from build123d import *

# Parameters (mm, degrees)
F0_W     = 20
F0_H     = 10.1
F1_DEPTH = 1.5
F2_R     = 1.1
F3_DEPTH = 1.5
F4_R     = 1


with BuildPart() as f1:
    # F0 (on Front) → F1 (new body)
    with BuildSketch(Plane.XZ):
        with Locations((10, 5.05)):
            Rectangle(F0_W, F0_H)
    extrude(amount=F1_DEPTH)

    # F2 (on face) → F3 (cut, through all)
    with BuildSketch(Plane.XZ.offset(1.5)):
        with Locations((2.3, 7.9)):
            Circle(F2_R)
        with Locations((17.7, 7.9)):
            Circle(F2_R)
        with Locations((2.3, 2.2)):
            Circle(F2_R)
        with Locations((17.7, 2.2)):
            Circle(F2_R)
        with BuildLine():
            Line((15.123475383, 10.1), (4.876524617, 10.1))
            ThreePointArc((4.876524617, 10.1), (10, 7.6), (15.123475383, 10.1))
        make_face()
        with BuildLine():
            ThreePointArc((15.123475383, 0), (10, 2.5), (4.876524617, 0))
            Line((4.876524617, 0), (15.123475383, 0))
        make_face()
    extrude(amount=-F3_DEPTH, mode=Mode.SUBTRACT)

    # F4
    f4_edges = [f1.edges().sort_by_distance(p)[0] for p in [
        (20, -0.75, 10.1),
        (20, -0.75, 0),
        (0, -0.75, 10.1),
        (0, -0.75, 0),
        (4.876525, -0.75, 10.1),
        (15.123475, -0.75, 10.1),
        (4.876525, -0.75, 0),
        (15.123475, -0.75, 0),
    ]]
    fillet(f4_edges, radius=F4_R)


solid = f1.part
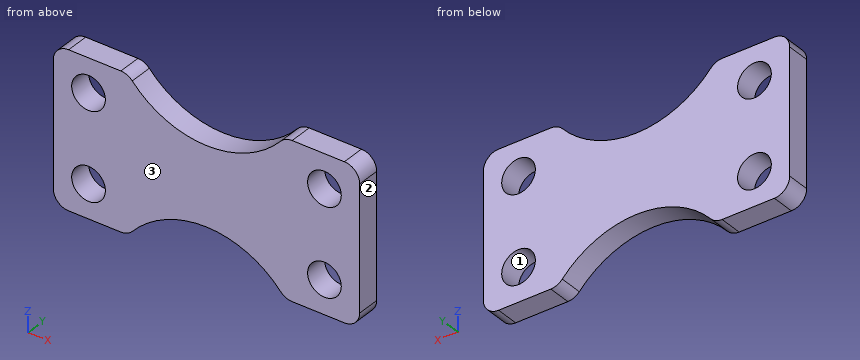
For this review, take the finished solid that the model builds, in its own axes (mm). Face numbers are marked on the shaded views. Give positions to 0.01 mm unless a question says otherwise; leave off trailing zeros. Order: outer loops, then holes, each group sorted by start corner. A loop starts at its lowest first (then second) coordinate and runs counter-clockwise, first axis right, second up. Notation, with made-up numbers: (13.5, 71.5) - (30.5, 71.5) arc R16 cw to (30.5, 83.5) - close; hole circle Ø3 at (37.5, 51). An arc over 180 degrees is marked (long way). Answer as a JSON object with one key per item and string values. Group by question number.
Item 1: Take a section at D-D on z = 7. Give the boundary of the cut face in (x, y), and give its area (3 significant figures).
Item 2: Take a section at B-B on z = 8.25. Give the boundary of the cut face in (x, y), and give its area (3 significant figures).
Item 3: Draft analysis for pull direction X (two halves, no side actions). For the marked faces 1, 2 and 3, state which applies: pulls with the +X half, pulls with the -X half, needs draft (parallel to the pull), parting line crosses it, or undercut.
Item 4: Take a section at A-A on x = 2.3. Give the boundary of the cut face in (y, z).
Item 5: Take a section at C-C on y = -1.15. Give the boundary of the cut face in (x, z).
Item 6: Wall thickness on line 1 along Z through (x, y) = (17.7, -1.2); line 2 along X through (y, z) = (-0.65, 2); line 3 along X through (y, z) = (-0.7, 1.5): over which ranges is each line inside the solid? List them lowest first.
Item 7: Clearance check with a flat-ended pin moving along its axis: pin 1 Ø2.5 at (x, z) = (17.7, 7.9) entering from +Y. State where the tip first meets the part, or that it passes through.
Reported:
{
 "1": {"outline": "(0, -1.5) - (1.67, -1.5) - (1.67, 0) - (0, 0) - close; (2.93, -1.5) - (17.07, -1.5) - (17.07, 0) - (2.93, 0) - close; (18.33, -1.5) - (20, -1.5) - (20, 0) - (18.33, 0) - close", "area": "26.2 mm^2"},
 "2": {"outline": "(0, -1.5) - (1.26, -1.5) - (1.26, 0) - (0, 0) - close; (3.34, -1.5) - (7.17, -1.5) - (7.17, 0) - (3.34, 0) - close; (12.83, -1.5) - (16.66, -1.5) - (16.66, 0) - (12.83, 0) - close; (18.74, -1.5) - (20, -1.5) - (20, 0) - (18.74, 0) - close", "area": "15.2 mm^2"},
 "3": {"face 1": "undercut", "face 2": "pulls with the +X half", "face 3": "needs draft"},
 "4": {"outline": "(-1.5, 0) - (0, 0) - (0, 1.1) - (-1.5, 1.1) - close; (-1.5, 3.3) - (0, 3.3) - (0, 6.8) - (-1.5, 6.8) - close; (-1.5, 9) - (0, 9) - (0, 10.1) - (-1.5, 10.1) - close"},
 "5": {"outline": "(0, 1) arc R1 ccw to (1, 0) - (4.41, 0) arc R1 ccw to (5.16, 0.33) arc R6.5 cw to (14.84, 0.33) arc R1 ccw to (15.59, 0) - (19, 0) arc R1 ccw to (20, 1) - (20, 9.1) arc R1 ccw to (19, 10.1) - (15.59, 10.1) arc R1 ccw to (14.84, 9.77) arc R6.5 cw to (5.16, 9.77) arc R1 ccw to (4.41, 10.1) - (1, 10.1) arc R1 ccw to (0, 9.1) - close; hole circle Ø2.2 at (2.3, 2.2); hole circle Ø2.2 at (2.3, 7.9); hole circle Ø2.2 at (17.7, 2.2); hole circle Ø2.2 at (17.7, 7.9)"},
 "6": {"line 1": "0 to 1.1, 3.3 to 6.8, 9 to 10.1", "line 2": "0 to 1.22, 3.38 to 7.5, 12.5 to 16.62, 18.78 to 20", "line 3": "0 to 1.45, 3.15 to 6.54, 13.46 to 16.85, 18.55 to 20"},
 "7": {"pin 1": "y = 0"}
}
